The figure shows three views and two pictorial views of one solid part (mm, origin at its lowest corner). Answer the questions. Round coordinates to 2 decimals unless told otherwise and drop trailing zeros. Order: outer loops, then holes, each group sorted by start corner. A loop starts at its lowest first (then second) coordinate and runs counter-clockwise, first axis right, second up.
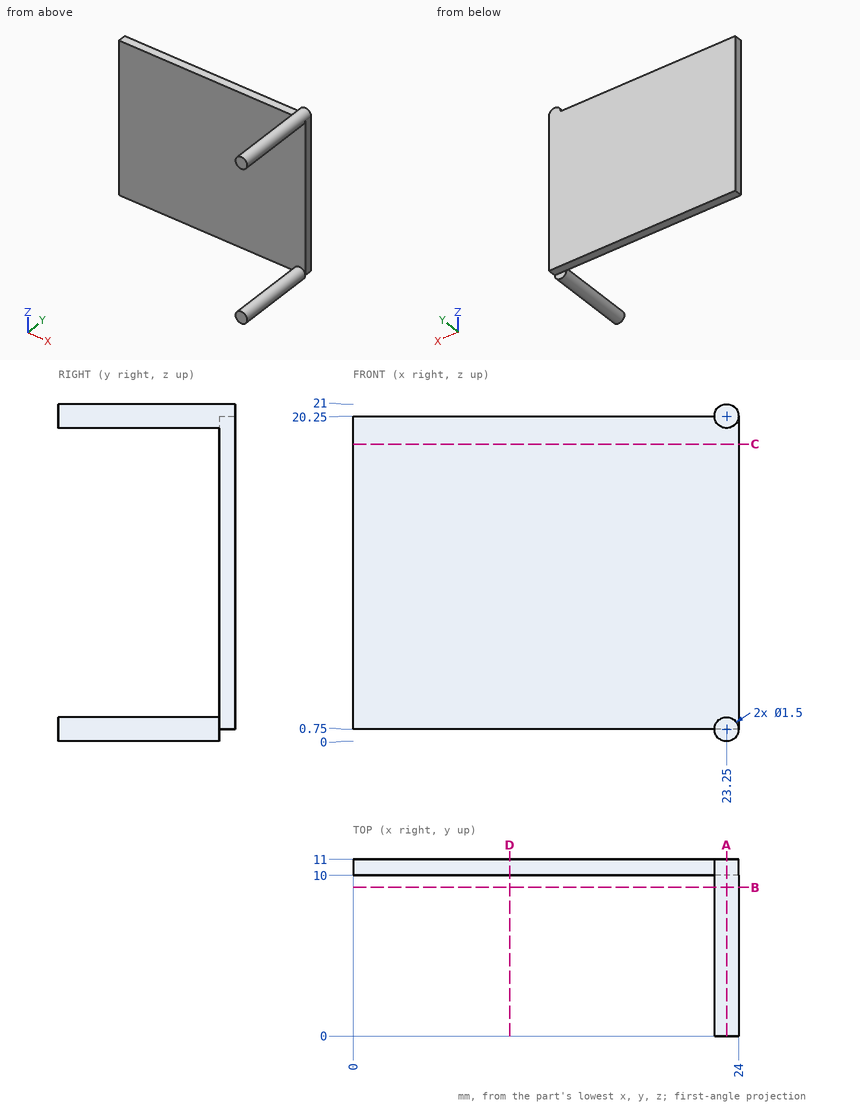
Item 1: Find section B-B (y = 9.25). Write down the section's boundary in (x, z).
Item 2: Find section A-A (x = 23.25). Write down the section's boundary in (y, z), plus the area to 4 significant figures.
Item 3: Find section D-D (x = 9.75). Write down the section's boundary in (y, z), plus the area to 3 significant figures.
Item 4: Find the intervals of material crossed by line 1 along Y through (x, z) = (13.5, 15.5), in increasing order.
Item 5: Given pin 1 (12 mm diameter, centred on x = 17.5, z = 8, fed in from -Y); pin 2 (1.1 mm diameter, centred on x = 12.5, y = 10.5, fed in from -Z), each flat-ended and moving along its own axis, determine where each tip first touches the part or whether it passes through.
Item 6: Find section C-C (z = 18.5). Write down the section's boundary in (x, y), plus the area to 3 significant figures.
Model answer:
1. outline: circle Ø1.5 at (23.25, 0.75); circle Ø1.5 at (23.25, 20.25)
2. outline: (0, 0) - (10, 0) - (10, 0.75) - (11, 0.75) - (11, 21) - (0, 21) - (0, 19.5) - (10, 19.5) - (10, 1.5) - (0, 1.5) - close
2. area: 50.25 mm2
3. outline: (10, 0.75) - (11, 0.75) - (11, 20.25) - (10, 20.25) - close
3. area: 19.5 mm2
4. line 1: y = 10 to 11
5. pin 1: stops at y = 10
5. pin 2: stops at z = 0.75
6. outline: (0, 10) - (24, 10) - (24, 11) - (0, 11) - close
6. area: 24.0 mm2
